The listing builds one solid part. Answer for the finished solid, in the listing's coordinates (mm). Coordinates: 2 decimals unless noted, no trailing zeros. Order: outer loops, then holes, each group sorted by start corner. A loop starts at its lowest first (then second) coordinate and runs counter-clockwise, first axis right, second up. Notation, with made-up numbers: (-13, 34.25) -> (37, 34.25) arc R27 cw to (37, 51.25) -> close; hole circle Ø7 at (45, -33.5). An arc over 180 degrees is marked (long way). Return JSON: item names as keys, results as strings.
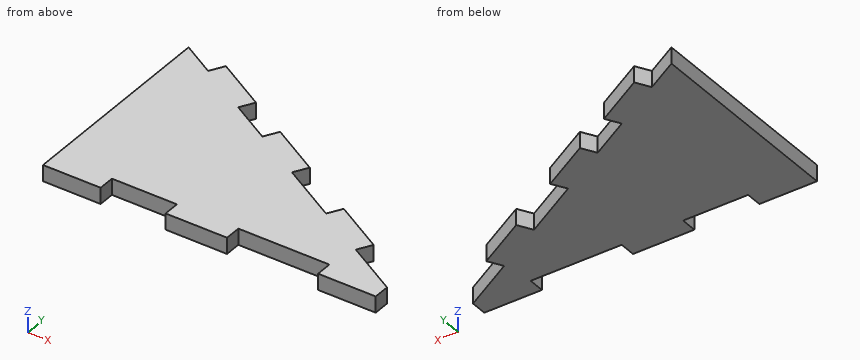
```python
from build123d import *

# Parameters (mm, degrees)
SKETCH1_W           = 109.982
SKETCH1_H           = 63.5
BOSS_EXTRUDE1_DEPTH = 5.334
CUT_EXTRUDE1_DEPTH  = 128.109173076
SKETCH7_W           = 19.05
SKETCH7_H           = 5.334
SKETCH7_W_2         = 20.295839927
BOSS_EXTRUDE4_DEPTH = 5.334
SKETCH9_W           = 19.270046927
SKETCH9_H           = 5.334
SKETCH9_W_2         = 18.946166646
SKETCH9_W_3         = 19.104051368
BOSS_EXTRUDE6_DEPTH = 5.334


with BuildPart() as part:
    # Sketch1 → Boss-Extrude1 (new body)
    with BuildSketch(Plane.XY):
        with Locations((54.991, 31.75)):
            Rectangle(SKETCH1_W, SKETCH1_H)
    extrude(amount=BOSS_EXTRUDE1_DEPTH)

    # Sketch2 → Cut-Extrude1 (cut, through all)
    with BuildSketch(Plane.XY.offset(5.334)):
        Polygon((0, 63.5), (109.982, 0), (109.982, 63.5), align=None)
    extrude(amount=-CUT_EXTRUDE1_DEPTH, mode=Mode.SUBTRACT)

    # Sketch7 → Boss-Extrude4 (add)
    with BuildSketch(Plane(origin=(0, 0, 0), x_dir=(-1, 0, 0), z_dir=(0, -1, 0))):
        with Locations((-9.525, -2.667)):
            Rectangle(SKETCH7_W, SKETCH7_H)
        with Locations((-50.685821834, -2.667)):
            Rectangle(SKETCH7_W_2, SKETCH7_H)
        with Locations((-100.457, -2.667)):
            Rectangle(SKETCH7_W, SKETCH7_H)
    extrude(amount=BOSS_EXTRUDE4_DEPTH)

    # Sketch9 → Boss-Extrude6 (add)
    with BuildSketch(Plane(origin=(27.496709855, 47.624301469, 0), x_dir=(0.866019052628739, -0.5000110003630135, 0), z_dir=(0.5000110003630134, 0.8660190526287389, 0))):
        with Locations((-9.635023464, -2.667)):
            Rectangle(SKETCH9_W, SKETCH9_H)
        with Locations((24.937675247, -2.667)):
            Rectangle(SKETCH9_W_2, SKETCH9_H)
        with Locations((65.750875897, -2.667)):
            Rectangle(SKETCH9_W_3, SKETCH9_H)
    extrude(amount=BOSS_EXTRUDE6_DEPTH)


solid = part.part
```
Item 1: Find the intervals of material crossed by probe 1 along X at (y, z) = (-1, 4.2); probe 2 along X at (y, z) = (35, 4.6); probe 3 along X at (y, z) = (22, 2.1), in increasing order.
Answer list:
{"probe 1": "0 to 19.05, 40.54 to 60.83, 90.93 to 109.98", "probe 2": "0 to 59.94", "probe 3": "0 to 71.88, 77.6 to 82.55"}
Item 2: The part is cut by section D-D on y = 12. Determine the outline of the cut face in (x, z).
Answer list:
{"outline": "(0, 0) -> (93.88, 0) -> (93.88, 5.33) -> (0, 5.33) -> close"}
Item 3: The part is cut by section B-B on y = 42.5. Determine the outline of the cut face in (x, z), plus the area to 3 significant figures.
Answer list:
{"outline": "(0, 0) -> (36.37, 0) -> (36.37, 5.33) -> (0, 5.33) -> close; (42.4, 0) -> (47.04, 0) -> (47.04, 5.33) -> (42.4, 5.33) -> close", "area": "219 mm2"}
Item 4: The part is cut by section C-C on x = 36.5. Determine the outline of the cut face in (y, z).
Answer list:
{"outline": "(0, 0) -> (42.43, 0) -> (42.43, 5.33) -> (0, 5.33) -> close"}
Item 5: Flat-ended cylindrical pins translate along their axes: pin 1 (10 mm diameter, centred on x = 49.5, y = 34.5, fed in from -Z); pin 2 (3 mm diameter, centred on y = 10.5, z = 4.5, fed in from +X); pin 3 (2 mm diameter, centred on x = 71.5, z = 4.5, fed in from +Y); pin 4 (2.5 mm diameter, centred on x = 69.5, z = 1.5, fed in from -Y). Find the tip coordinate at first contact, or state that the pin passes through.
Answer list:
{"pin 1": "z = 0", "pin 2": "x = 94.39", "pin 3": "y = 22.8", "pin 4": "y = 0"}
Item 6: The part is cut by section A-A on z = 1.25. Determine the outline of the cut face in (x, y).
Answer list:
{"outline": "(0, -5.33) -> (19.05, -5.33) -> (19.05, 0) -> (40.54, 0) -> (40.54, -5.33) -> (60.83, -5.33) -> (60.83, 0) -> (90.93, 0) -> (90.93, -5.33) -> (109.98, -5.33) -> (109.98, 0) -> (92.71, 9.97) -> (95.38, 14.59) -> (78.83, 24.14) -> (76.17, 19.52) -> (57.3, 30.42) -> (59.96, 35.04) -> (43.56, 44.51) -> (40.89, 39.89) -> (27.5, 47.62) -> (30.16, 52.24) -> (13.48, 61.88) -> (10.81, 57.26) -> (0, 63.5) -> close"}
